Check sheet for the drawn part. Datum: minimum x, y, z corner. Units: mm. Coordinates: 2 decimals unless noted, no trailing zeros. Write each loop counter-clockwise with the first axis right and the second up, starting at its lowest first coordinate (ties: lowest second). Pieces come first, ordered by that corner, then holes. Notation, with made-up numbers: (82.5, 2.5) - (133.5, 2.5) arc R13 ccw to (133.5, 21.5) - close; hole circle Ø11 at (-20, 41). An arc over 180 degrees is marked (long way). Use one line per item in the form item = value. Start each with the question number.
1. Scan lines: line 1 along X through (y, z) = (5.25, 6); line 2 along Y through (x, z) = (88, 3.7); line 3 along Y through (x, z) = (22, 2.15). Record each from-to range of solid material in increasing order.
2. Cross-section at A-A on x = 22. Record the boundary of the cut face in (y, z).
3. Go/stop test with flat-tipped pins: pin 1 Ø10 at (x, y) = (39, 94) entering from +Z; pin 2 Ø1.8 at (x, y) = (79, 35) entering from +Z. Record where each tip stops, or that it passes through.
4. Cross-section at D-D on x = 63. Record the boundary of the cut face in (y, z).
5. Draft check along Y on the marked faces 1, 2, 3 and 4. Enter one of: +Y half, -Y half, draft (parallel to the pull), parting line (faces both ways), or undercut.
6. Cross-section at C-C on x = 39. Record the boundary of the cut face in (y, z), then the cut area to 3 significant figures.
7. Cross-section at B-B on y = 67. Record the boundary of the cut face in (x, z), then the cut area to 3 significant figures.
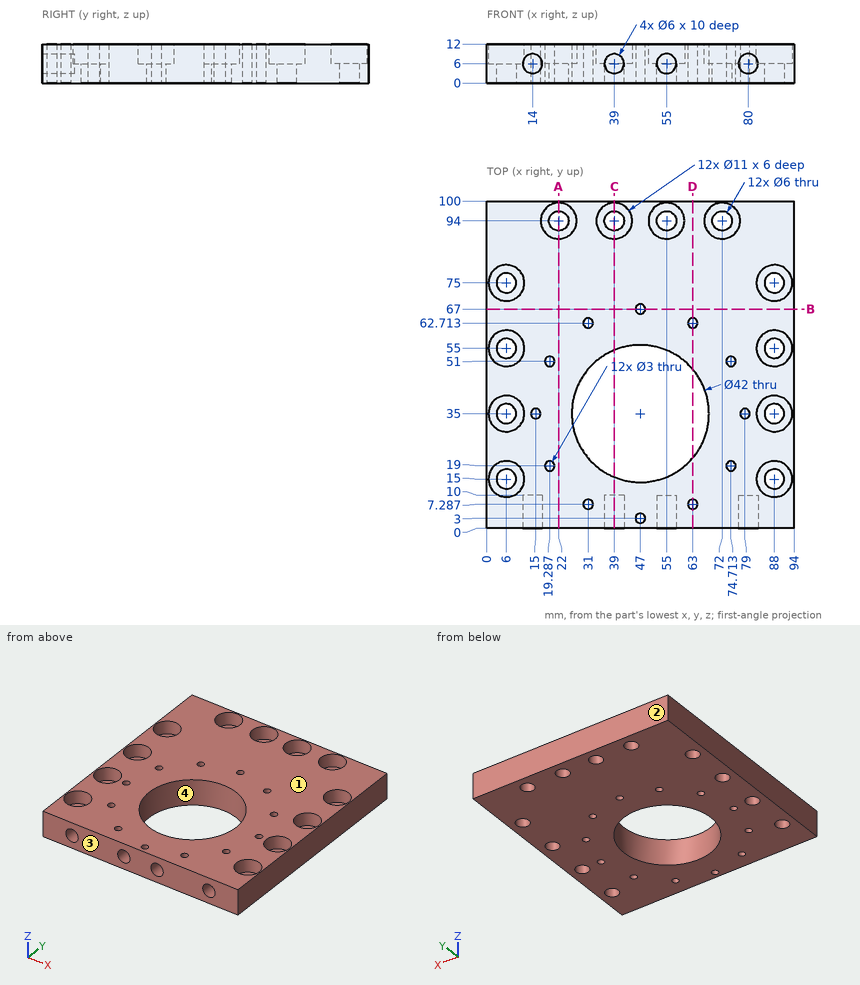
Final values:
q1.line_1 = 0 to 11, 17 to 36, 42 to 52, 58 to 77, 83 to 94
q1.line_2 = 0 to 12, 18 to 32, 38 to 52, 58 to 72, 78 to 100
q1.line_3 = 0 to 91, 97 to 100
q2.outline = (0, 0) - (91, 0) - (91, 6) - (88.5, 6) - (88.5, 12) - (0, 12) - close; (97, 0) - (100, 0) - (100, 12) - (99.5, 12) - (99.5, 6) - (97, 6) - close
q3.pin_1 = 6
q3.pin_2 = through
q4.outline = (0, 0) - (5.79, 0) - (5.79, 12) - (0, 12) - close; (8.79, 0) - (21.4, 0) - (21.4, 12) - (8.79, 12) - close; (48.6, 0) - (61.21, 0) - (61.21, 12) - (48.6, 12) - close; (64.21, 0) - (100, 0) - (100, 12) - (64.21, 12) - close
q5.face_1 = draft
q5.face_2 = +Y half
q5.face_3 = -Y half
q5.face_4 = undercut
q6.outline = (0, 0) - (15.58, 0) - (15.58, 12) - (0, 12) - (0, 9) - (10, 9) - (10, 3) - (0, 3) - close; (54.42, 0) - (91, 0) - (91, 6) - (88.5, 6) - (88.5, 12) - (54.42, 12) - close; (97, 0) - (100, 0) - (100, 12) - (99.5, 12) - (99.5, 6) - (97, 6) - close
q6.area = 572 mm²
q7.outline = (0, 0) - (45.5, 0) - (45.5, 12) - (0, 12) - close; (48.5, 0) - (94, 0) - (94, 12) - (48.5, 12) - close
q7.area = 1,090 mm²
